For this review, use the dimensioned drawing (mm, ordinates from the lowest corner) and the shaded views. A direction names the side the tool comes from. Round coordinates to 2 decimals unless told otherwise and drop trailing zeros. Order: outer loops, then holes, each group sorted by start corner. A loop starts at its lowest first (then second) coordinate and runs counter-clockwise, first axis right, second up. Notation, with made-up numbers: (72.5, -39.75) - (104.5, -39.75) arc R36 cw to (104.5, -3.75) - close; hole circle Ø9 at (-1.5, 43.25). An arc over 180 degrees is marked (long way). Write item = value, one per line.
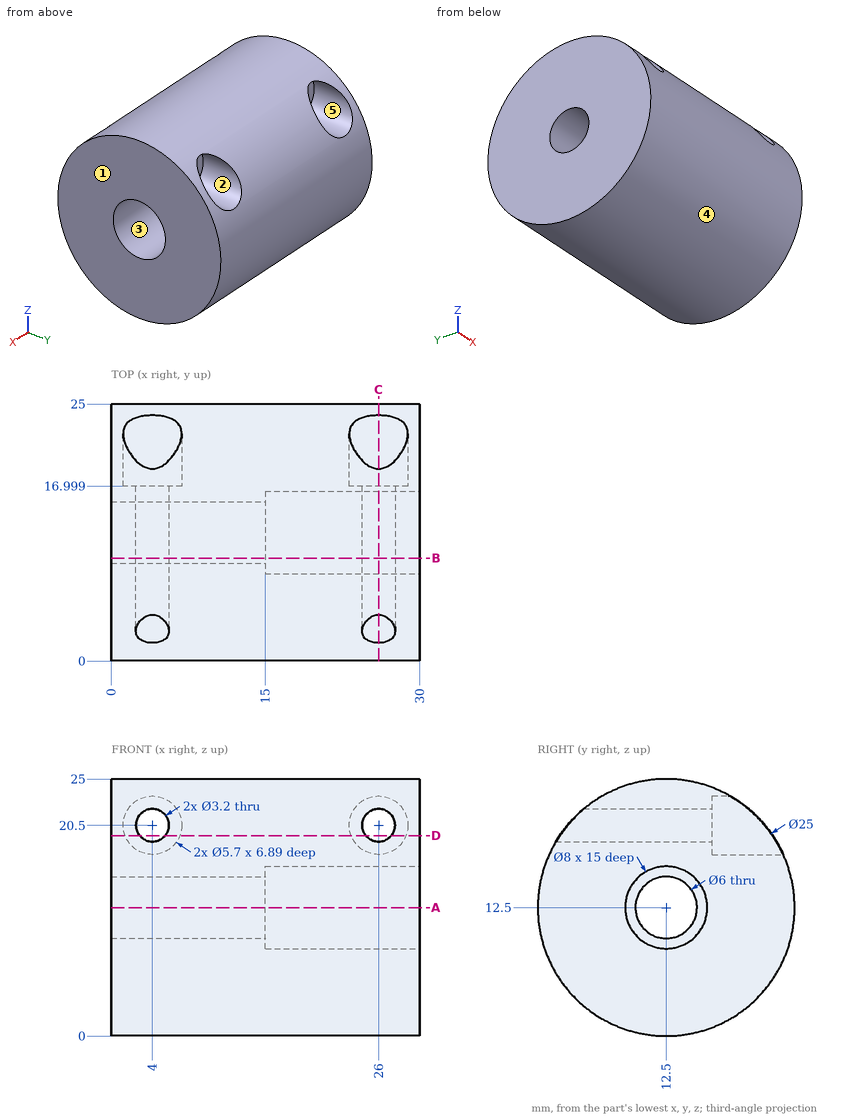
Item 1: Take a section at D-D, the plane z = 19.5. State the section outline as (x, y) points.
Data:
outline = (0, 2.14) - (2.75, 2.14) - (2.75, 17) - (1.33, 17) - (1.33, 22.86) - (0, 22.86) - close; (5.25, 2.14) - (24.75, 2.14) - (24.75, 17) - (23.33, 17) - (23.33, 22.86) - (6.67, 22.86) - (6.67, 17) - (5.25, 17) - close; (27.25, 2.14) - (30, 2.14) - (30, 22.86) - (28.67, 22.86) - (28.67, 17) - (27.25, 17) - close
Item 2: Take a section at C-C, the plane x = 26. Count the separate pieces of the cut face and the enclosed holes in it, and give its area (3 significant figures).
Data:
separate_pieces = 2
enclosed_holes = 1
area = 368 mm2
Item 3: Insertion check: P1, Ø3, axis at x = 26, z = 19.5, coming from the +Y side; P2, Ø3, axis at x = 18.5, z = 10, coming from the -Y side; P3, Ø5, axis at x = 26, z = 20.5, coming from the -Y side (1 decimal). Each pin has a flat end and moves straight along its axis. Give the tip position at first contact, or say it passes through.
Data:
P1 = 17
P2 = 0.04
P3 = 1.3
Item 4: Take a section at B-B, the plane y = 10. State the section outline as (x, z) points, and give its area (3 significant figures).
Data:
outline = (0, 0.25) - (30, 0.25) - (30, 9.38) - (15, 9.38) - (15, 10.84) - (0, 10.84) - close; (0, 14.16) - (15, 14.16) - (15, 15.62) - (30, 15.62) - (30, 24.75) - (0, 24.75) - close; hole circle Ø3.2 at (4, 20.5); hole circle Ø3.2 at (26, 20.5)
area = 575 mm2
Item 5: The part is to be moulded in two halves that separate along X. For the marked faces 1, 2 and 3, say which applies: +X half, -X half, draft (parallel to the pull), parting line (faces both ways), or undercut.
Data:
face_1 = +X half
face_2 = undercut
face_3 = draft
Item 6: For line 1 along Y through (x, z) = (26.75, 12.5); line 2 along Z through (x, y) = (26, 14.5) (1 decimal); line 3 along Y through (x, z) = (3.5, 12.5), list the stretches that pass through material, from the lowest coordinate up. Write a range as [from, to].
Data:
line_1 = [0, 8.5], [16.5, 25]
line_2 = [0.2, 9], [16, 18.9], [22.1, 24.8]
line_3 = [0, 9.5], [15.5, 25]
Item 7: Take a section at A-A, the plane z = 12.5. State the section outline as (x, y) points, and give its area (3 significant figures).
Data:
outline = (0, 0) - (30, 0) - (30, 8.5) - (15, 8.5) - (15, 9.5) - (0, 9.5) - close; (0, 15.5) - (15, 15.5) - (15, 16.5) - (30, 16.5) - (30, 25) - (0, 25) - close
area = 540 mm2
Item 8: For the marked faces 4 and 5, list the 3-axis set-ups (+Z, -Z, +X, -X, +Y, -Y) from which the entire face can be reached by the end or side of a thin tool; tool diameter is ignored.
Data:
face_4 = +X, -X
face_5 = +Y
